Could you check a few things on this model? Use its own coordinates, in mm. Face numbers are marked on the shaded views. A direction names the side the tool comes from. Give positions to 0.01 mm unless a question says otherwise; leave off trailing zeros. Loops run counter-clockwise (first coordinate to the right, second up) from the corner with the lowest first, then second, coordinate; pieces in that order, holes last. Notation, with made-up numbers: (-35, -6.5) -> (-16, -6.5) arc R20 ccw to (-16, 26.5) -> close; hole circle Ø11 at (23.5, 47). An arc over 180 degrees is marked (long way). Write each question's results on one line, items separated by ' | '. Start each with the question number.
Q1. Will these pins go through, and if not, where does the flat tip stop? P1, Ø1, axis at x = -8.5, y = 5, coming from the -Z side; P2, Ø8, axis at x = -11.5, y = -14.5, coming from the +Z side; P3, Ø5, axis at x = -12, y = -1.5, coming from the +Z side.
Q2. If I drill on line 1 along Z through (x, y) = (3, -14.5); line 2 along Z through (x, y) = (7.5, -8); line 3 along Y through (x, z) = (18.5, 23.5), over which ranges is the centre line in solid material (lowest first)?
Q3. If we section it at B-B, the plane y = 0: List the corners of the cut face in (x, z) for me.
Q4. Which directions (+Z, -Z, +X, -X, +Y, -Y) give clear straight access to the entire face, cutting with the end or side of a thin tool? Please do the marked faces 1 and 2.
Q5. If we section it at D-D, the plane y = 4.5: List the corners of the cut face in (x, z) for me, plus the area to 3 significant figures.
Q6. If we section it at A-A, the plane z = 31.5: List the corners of the cut face in (x, y) for me.
Q7. We'd pull the mould along Y, two halves only. Please class the marked faces 3, 4 and 5: released by +Y, released by -Y, zero draft, split by the parting line, or undercut.
from build123d import *

# Parameters (mm, degrees)
F0_W     = 42
F0_H     = 42
F1_DEPTH = 40
F2_R     = 11
F3_DEPTH = 2
F4_R     = 2.5
F5_DEPTH = 20
F6_SIZE  = 5


with BuildPart() as f1:
    # F0 (on Top) → F1 (new body)
    with BuildSketch(Plane.XY):
        Rectangle(F0_W, F0_H)
    extrude(amount=F1_DEPTH)

    # F2 (on face) → F3 (join)
    with BuildSketch(Plane.XY.offset(40)):
        Circle(F2_R)
    extrude(amount=F3_DEPTH)

    # F4 (on face) → F5 (join)
    with BuildSketch(Plane.XY.offset(42)):
        Circle(F4_R)
    extrude(amount=F5_DEPTH)

    # F6
    f6_edges = [f1.edges().sort_by_distance(p)[0] for p in [
        (21, -21, 20),
        (-21, 21, 20),
        (-21, -21, 20),
        (21, 21, 20),
    ]]
    chamfer(f6_edges, length=F6_SIZE)


solid = f1.part
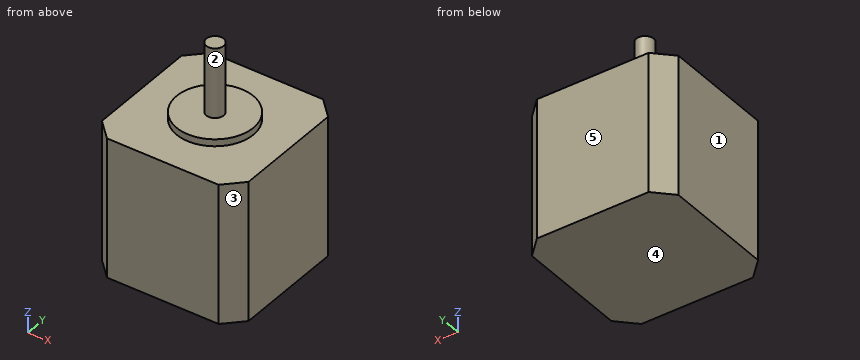
Final values:
1) P1: stops at z = 0 | P2: stops at z = 40 | P3: stops at z = 42
2) line 1: z = 0 to 40 | line 2: z = 0 to 42 | line 3: y = -18.5 to 18.5
3) outline: (-21, 0) -> (21, 0) -> (21, 40) -> (11, 40) -> (11, 42) -> (2.5, 42) -> (2.5, 62) -> (-2.5, 62) -> (-2.5, 42) -> (-11, 42) -> (-11, 40) -> (-21, 40) -> close
4) face 1: +Z, -Z, -X, +Y, -Y | face 2: +Z
5) outline: (-21, 0) -> (21, 0) -> (21, 40) -> (10.04, 40) -> (10.04, 42) -> (-10.04, 42) -> (-10.04, 40) -> (-21, 40) -> close | area: 1,720 mm²
6) outline: (-21, -16) -> (-16, -21) -> (16, -21) -> (21, -16) -> (21, 16) -> (16, 21) -> (-16, 21) -> (-21, 16) -> close
7) face 3: released by -Y | face 4: zero draft | face 5: released by +Y
